Design review of the part shown in the three views and the two pictorial views. Dimensions are in mm from the part's minimum x, y and z. Give positions to 0.01 mm unless a question says otherwise; leave off trailing zeros. Put each result on its own line as item: value.
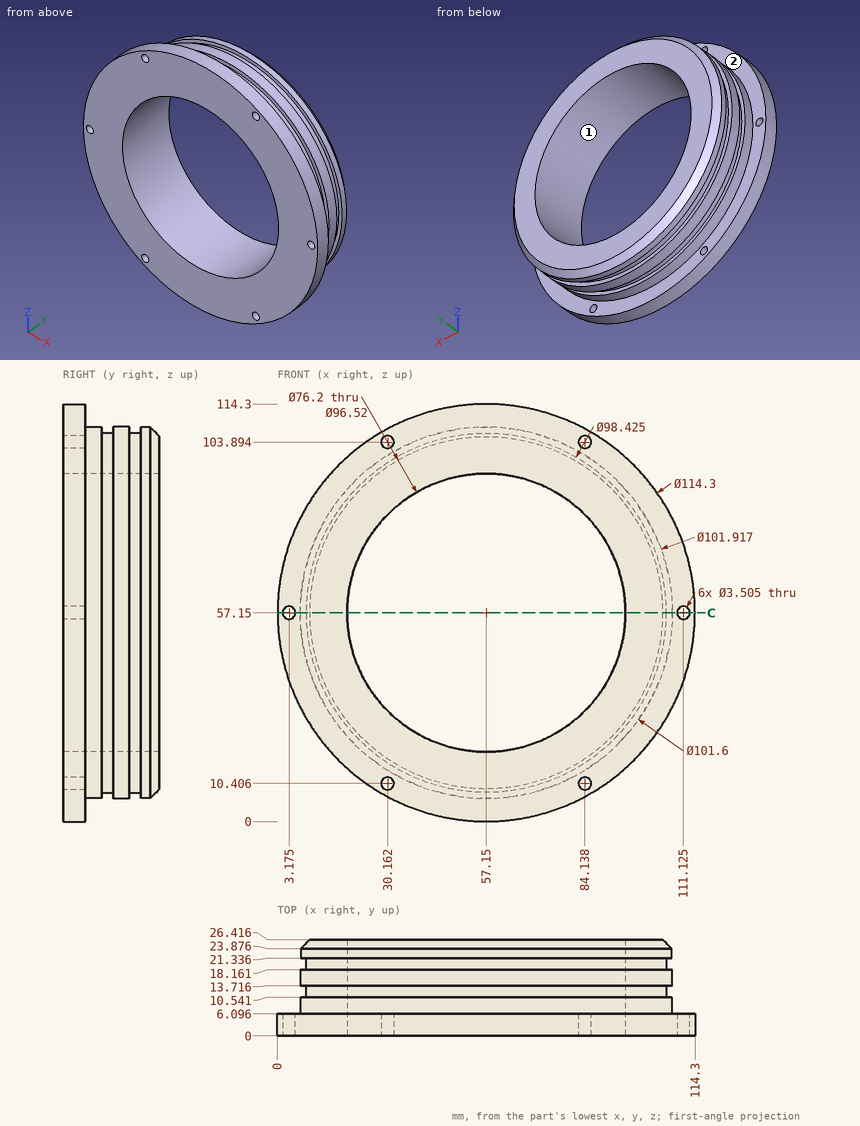
(1) The part is to be moulded in two halves that separate along X. For the marked faces 1 and 2, say which applies: pulls with the +X half, pulls with the -X half, needs draft (parallel to the pull), parting line crosses it, or undercut.
The answers:
face 1: undercut
face 2: needs draft
(2) Take a section at C-C, the plane z = 57.15. Count the separate pieces of the cut face and the enclosed holes in it.
The answers:
separate pieces: 4
enclosed holes: 0
(3) Clearance check with flat-ended pins moving along their axes: pin 1 Ø10 at (y, z) = (8, 41.5) entering from -X; pin 2 Ø4 at (x, y) = (37.5, 22.5) entering from -Z (1 decimal); pin 3 Ø10 at (x, y) = (40, 16.5) entering from +Z; pin 4 Ø2 at (x, z) = (30.16, 103.89) entering from -Y. State where each tip first meets the part, or that it passes through.
The answers:
pin 1: x = 1.07
pin 2: z = 9.5
pin 3: z = 106.64
pin 4: through
(4) Wall thickness on L1, parallel to Z at x = 57.15, y = 16.5; L2, parallel to Z at x = 29, y = 17.5 (1 decimal); L3, parallel to X at y = 6.75, z = 91.5 (1 decimal): over which ranges is each line inside the solid? List them lowest first.
The answers:
L1: 6.19 to 19.05, 95.25 to 108.11
L2: 14.7 to 31.5, 82.8 to 99.6
L3: 19.7 to 40.7, 73.6 to 94.6
